Geometry check sheet. Reference: the model listing, model coordinates, mm. Face numbers are marked on the shaded views. A direction names the side the tool comes from. Round coordinates to 2 decimals unless told otherwise and drop trailing zeros. Write each loop counter-clockwise with the first axis right and the second up, starting at its lowest first coordinate (ties: lowest second). Pieces come first, ordered by that corner, then holes.
Item 1: Draft check along Y on the marked faces 1, 2, 3 and 4. Enter one of: pulls with the +Y half, pulls with the -Y half, needs draft (parallel to the pull), parting line crosses it, or undercut.
Item 2: Cross-section at B-B (z = 10.75). Enter the section's corners in (x, y).
Item 3: Access from +Z, -Z, +X, -X, +Y, -Y to the whole of each face (thin tool, end or side, straight path). Record for the marked faces 5, 6 and 7.
Item 4: Depth check by flat-ended pin: P1, Ø1, axis at x = -12, z = 1.5, coming from the +Y side; P2, Ø10, axis at x = 1, y = -3.5, coming from the +Z side; P3, Ø6, axis at x = -15.5, z = 7.5, coming from the -Y side. Enter the tip coordinate at first touch or a pass-through.
Item 5: Scan lines: probe 1 along Y at (x, z) = (-13, 4.25); probe 2 along Y at (x, z) = (-7.5, 8.5); probe 3 along Z at (x, y) = (-14.5, -1.75). Record each from-to range of solid material in increasing order.
Item 6: Cross-section at A-A (x = -13). Enter the section's corners in (y, z).
Item 7: Cross-section at C-C (y = -8). Enter the section's corners in (x, z), then the cut area to 3 significant figures.
from build123d import *

# Parameters (mm, degrees)
F1_DEPTH = 12
F2_DEPTH = 0.6


with BuildPart() as f1:
    # F0 (on Top) → F1 (new body)
    with BuildSketch(Plane.XY):
        with BuildLine():
            ThreePointArc((-11.6743308159, 5), (-11.3948589306, 5.6077794136), (-11.0837719211, 6.2))
            Line((-11.0837719211, 6.2), (-24.2, 6.2))
            Line((-24.2, 6.2), (-24.2, 0))
            Line((-24.2, 0), (-24.2, -6.2))
            Line((-24.2, -6.2), (-11.0837719211, -6.2))
            ThreePointArc((-11.0837719211, -6.2), (-11.3948589306, -5.6077794136), (-11.6743308159, -5))
            Line((-11.6743308159, -5), (-23, -5))
            Line((-23, -5), (-23, 0))
            Line((-23, 0), (-23, 5))
            Line((-23, 5), (-11.6743308159, 5))
        make_face()
        with BuildLine():
            ThreePointArc((-9.6855562566, 6.2), (3.2300234557, 11.0370715534), (11.5, 0))
            ThreePointArc((11.5, 0), (3.2300234557, -11.0370715534), (-9.6855562566, -6.2))
            Line((-9.6855562566, -6.2), (-11.0837719211, -6.2))
            ThreePointArc((-11.0837719211, -6.2), (3.2035992728, -12.2893023276), (12.7, 0))
            ThreePointArc((12.7, 0), (3.2035992728, 12.2893023276), (-11.0837719211, 6.2))
            Line((-11.0837719211, 6.2), (-9.6855562566, 6.2))
        make_face()
        with BuildLine():
            ThreePointArc((-10.3561575886, 5), (-10.038803388, 5.610029103), (-9.6855562566, 6.2))
            Line((-9.6855562566, 6.2), (-11.0837719211, 6.2))
            ThreePointArc((-11.0837719211, 6.2), (-11.3948589306, 5.6077794136), (-11.6743308159, 5))
            Line((-11.6743308159, 5), (-10.3561575886, 5))
        make_face()
        with BuildLine():
            Line((-11.0837719211, -6.2), (-9.6855562566, -6.2))
            ThreePointArc((-9.6855562566, -6.2), (-10.038803388, -5.610029103), (-10.3561575886, -5))
            Line((-10.3561575886, -5), (-11.6743308159, -5))
            ThreePointArc((-11.6743308159, -5), (-11.3948589306, -5.6077794136), (-11.0837719211, -6.2))
        make_face()
    extrude(amount=F1_DEPTH)

    # F0 (on Top) → F2 (join)
    with BuildSketch(Plane.XY):
        with BuildLine():
            ThreePointArc((-9.6855562566, -6.2), (3.2300234557, -11.0370715534), (11.5, 0))
            ThreePointArc((11.5, 0), (3.2300234557, 11.0370715534), (-9.6855562566, 6.2))
            ThreePointArc((-9.6855562566, 6.2), (-10.038803388, 5.610029103), (-10.3561575886, 5))
            Line((-10.3561575886, 5), (0, 5))
            Line((0, 5), (0, 0))
            Line((0, 0), (-11.5, 0))
            ThreePointArc((-11.5, 0), (-11.2103927734, -2.5645845405), (-10.3561575886, -5))
            ThreePointArc((-10.3561575886, -5), (-10.038803388, -5.610029103), (-9.6855562566, -6.2))
        make_face()
        with BuildLine():
            ThreePointArc((-12.7, 0), (-12.4409405063, 2.5520578596), (-11.6743308159, 5))
            Line((-11.6743308159, 5), (-23, 5))
            Line((-23, 5), (-23, 0))
            Line((-23, 0), (-12.7, 0))
        make_face()
        with BuildLine():
            Line((0, 5), (-10.3561575886, 5))
            ThreePointArc((-10.3561575886, 5), (-11.2103927734, 2.5645845405), (-11.5, 0))
            Line((-11.5, 0), (0, 0))
            Line((0, 0), (0, 5))
        make_face()
        with BuildLine():
            ThreePointArc((-11.5, 0), (-11.2103927734, 2.5645845405), (-10.3561575886, 5))
            Line((-10.3561575886, 5), (-11.6743308159, 5))
            ThreePointArc((-11.6743308159, 5), (-12.4409405063, 2.5520578596), (-12.7, 0))
            Line((-12.7, 0), (-11.5, 0))
        make_face()
        with BuildLine():
            Line((-23, -5), (-11.6743308159, -5))
            ThreePointArc((-11.6743308159, -5), (-12.4409405063, -2.5520578596), (-12.7, 0))
            Line((-12.7, 0), (-23, 0))
            Line((-23, 0), (-23, -5))
        make_face()
        with BuildLine():
            Line((-11.6743308159, -5), (-10.3561575886, -5))
            ThreePointArc((-10.3561575886, -5), (-11.2103927734, -2.5645845405), (-11.5, 0))
            Line((-11.5, 0), (-12.7, 0))
            ThreePointArc((-12.7, 0), (-12.4409405063, -2.5520578596), (-11.6743308159, -5))
        make_face()
    extrude(amount=F2_DEPTH)


solid = f1.part
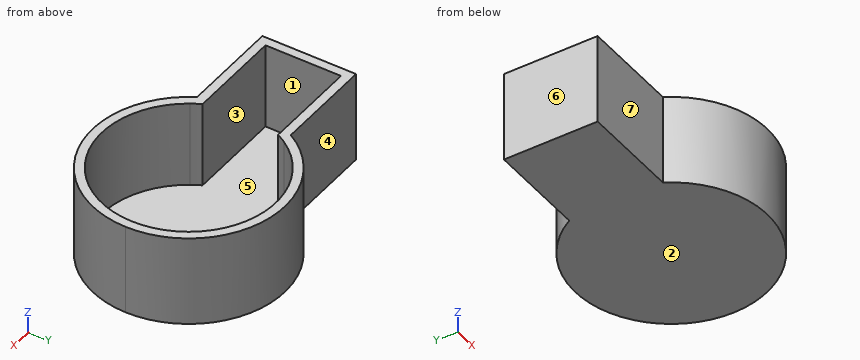
Resolved:
1. face 1: undercut
1. face 2: needs draft
1. face 3: undercut
1. face 4: pulls with the +Y half
2. outline: (-24.2, -6.2) - (-11.08, -6.2) arc R12.7 ccw (long way) to (-11.08, 6.2) - (-24.2, 6.2) - close; hole (-23, -5) - (-10.36, -5) arc R11.5 ccw (long way) to (-10.36, 5) - (-23, 5) - close
3. face 5: +Z
3. face 6: +Z, -Z, -X, +Y, -Y
3. face 7: +Z, -Z, -X, -Y
4. P1: stops at y = 6.2
4. P2: stops at z = 0.6
4. P3: stops at y = -6.2
5. probe 1: y = -6.2 to -5, 5 to 6.2
5. probe 2: y = -10.25 to -8.72, 8.72 to 10.25
5. probe 3: z = 0 to 0.6
6. outline: (-6.2, 0) - (6.2, 0) - (6.2, 12) - (5, 12) - (5, 0.6) - (-5, 0.6) - (-5, 12) - (-6.2, 12) - close
7. outline: (-9.86, 0) - (9.86, 0) - (9.86, 12) - (8.26, 12) - (8.26, 0.6) - (-8.26, 0.6) - (-8.26, 12) - (-9.86, 12) - close
7. area: 48.4 mm2
